Model file for the job. Use its own axes, mm. A direction names the side the tool comes from. Coordinates: 2 decimals unless noted, no trailing zeros. Order: outer loops, then holes, each group sorted by start corner. A loop starts at its lowest first (then second) coordinate and runs counter-clockwise, first axis right, second up.
from build123d import *

# Parameters (mm, degrees)
ESQUISSE2_R             = 3.2
BOSS_EXTRU_1_DEPTH      = 25
ESQUISSE3_R             = 2
ENL_V_MAT_EXTRU_1_DEPTH = 14
ESQUISSE4_R             = 1
ENL_V_MAT_EXTRU_2_DEPTH = 4


with BuildPart() as part:
    # Esquisse1 → Révolution2 (revolve)
    with BuildSketch(Plane.XY):
        Polygon((0, 0), (24.4, 0), (24.4, 6.8), (19.3, 6.8), (19.3, 11.85), (0, 11.85), align=None)
    revolve(axis=Axis((0, 0, 0), (1, 0, 0)))

    # Esquisse2 → Boss.-Extru.1 (add)
    with BuildSketch(Plane(origin=(0, 0, 0), x_dir=(1, 0, 0), z_dir=(0, 1, 0))):
        with Locations((7, 0)):
            Circle(ESQUISSE2_R)
    extrude(amount=BOSS_EXTRU_1_DEPTH)

    # Esquisse3 → Enlèv. mat.-Extru.1 (cut)
    with BuildSketch(Plane(origin=(24.4, 0, 0), x_dir=(0, 0, -1), z_dir=(1, 0, 0))):
        Circle(ESQUISSE3_R)
    extrude(amount=-ENL_V_MAT_EXTRU_1_DEPTH, mode=Mode.SUBTRACT)

    # Esquisse4 → Enlèv. mat.-Extru.2 (cut)
    with BuildSketch(Plane(origin=(19.3, 0, 0), x_dir=(0, 0, -1), z_dir=(1, 0, 0))):
        with Locations((0, -9.5)):
            Circle(ESQUISSE4_R)
        with Locations((-8.227241336, 4.75)):
            Circle(ESQUISSE4_R)
        with Locations((8.227241336, 4.75)):
            Circle(ESQUISSE4_R)
    extrude(amount=-ENL_V_MAT_EXTRU_2_DEPTH, mode=Mode.SUBTRACT)


solid = part.part
Q1. Probe line 1 (X direction, y = 9.5, z = -1.5); line 2 (Y direction, x = 14.25, z = -0.25); line 3 (Z direction, x = 19, y = 1.5). List the from-to ranges inside material, lowest first.
Established:
line 1: x = 0 to 19.3
line 2: y = -11.85 to -1.98, 1.98 to 11.85
line 3: z = -11.75 to -1.32, 1.32 to 11.75
Q2. Cut at A-A, the plane y = 0. List the corners of the cut face in (x, z).
Established:
outline: (0, -11.85) - (19.3, -11.85) - (19.3, -6.8) - (24.4, -6.8) - (24.4, -2) - (10.4, -2) - (10.4, 2) - (24.4, 2) - (24.4, 6.8) - (19.3, 6.8) - (19.3, 11.85) - (0, 11.85) - close
Q3. Which spindle directions (+Z, -Z, +X, -X, +Y, -Y) get a long thin tool onto all of the face, cutting with end or side? Do faces 1 (the face through (4.461, 18.104, 1.947)), 2 (the face through (17.33, -8.51, 0.13)), 3 (the face through (0, 0, 0)). Say none if no direction does.
Established:
face 1: +Y
face 2: +X
face 3: +Z, -Z, -X, +Y, -Y
Q4. Mould opens along Y. For faces 4 (the face through (17.328, 4.794, 9.226)), 5 (the face through (9.515, 11.303, 3.559)), 6 (the face through (19.3, -5, -5)) say: pulls with the +Y half, pulls with the -Y half, needs draft (parallel to the pull), parting line crosses it, or undercut.
Established:
face 4: undercut
face 5: parting line crosses it
face 6: needs draft
Q5. Cut at C-C, the plane z = 0. List the corners of the cut face in (x, y).
Established:
outline: (0, -11.85) - (19.3, -11.85) - (19.3, -10.5) - (15.3, -10.5) - (15.3, -8.5) - (19.3, -8.5) - (19.3, -6.8) - (24.4, -6.8) - (24.4, -2) - (10.4, -2) - (10.4, 2) - (24.4, 2) - (24.4, 6.8) - (19.3, 6.8) - (19.3, 11.85) - (10.2, 11.85) - (10.2, 25) - (3.8, 25) - (3.8, 11.85) - (0, 11.85) - close
Q6. Cut at D-D, the plane x = 12.5. List the corners of the cut face in (y, z).
Established:
outline: circle Ø23.7 at (0, 0); hole circle Ø4 at (0, 0)
Q7. Cut at B-B, the plane x = 17.5. List the corners of the cut face in (y, z).
Established:
outline: circle Ø23.7 at (0, 0); hole circle Ø2 at (-9.5, 0); hole circle Ø4 at (0, 0); hole circle Ø2 at (4.75, -8.23); hole circle Ø2 at (4.75, 8.23)
Q8. Drop flat-ended pins along their axis: P1, Ø1, axis at y = 4.5, z = 8, coming from the +X side; P2, Ø2.5, axis at y = 4.75, z = -8.23, coming from the -X side; P3, Ø1, axis at x = 4.5, y = 16, coming from the +Z side; P4, Ø4, axis at x = 18.5, z = -4, coming from the +Y side. Give the stop position or say it passes through.
Established:
P1: stops at x = 15.3
P2: stops at x = 0
P3: stops at z = 2.5
P4: stops at y = 11.68
